```python
from build123d import *

# Parameters (mm, degrees)
F1_DEPTH = 3
F2_D     = 4


with BuildPart() as f1:
    # F0 (on Top) → F1 (new body)
    with BuildSketch(Plane.XY):
        Polygon((-13.5, -20), (13.5, -20), (13.5, 20), (-13.5, 20), (-13.5, 0), (-55, 0), (-55, -4.7585600987), (-55, -20), align=None)
    extrude(amount=F1_DEPTH)

    # F2 (through all)
    with Locations(Plane(origin=(0, 0, 0), x_dir=(1, 0, 0), z_dir=(0, 0, -1))):
        with Locations((-51, 10), (-26, 10), (-10, 10), (10, -10), (10, 10), (-10, -10)):
            Hole(F2_D / 2)


solid = f1.part
```
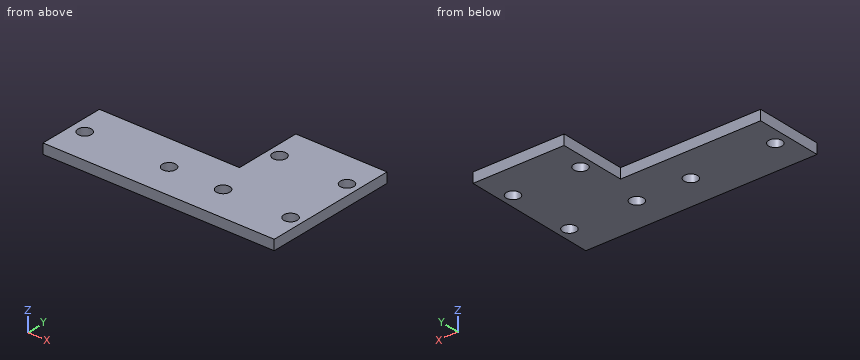
Work out the finished part from the listing and answer in its coordinate system (mm). Give positions to 0.01 mm unless a question says otherwise; leave off trailing zeros. Loops run counter-clockwise (first coordinate to the right, second up) from the corner with the lowest first, then second, coordinate; pieces in that order, holes last. Notation, with made-up numbers: M 2,-7 L 48,-7 A14 cw 48,-2 Z; hole C -12,-19.75 d4. An arc over 180 degrees is marked long. One line per item, written item: value. Start each with the question number.
1. Find section B-B (y = -10). Give the vertices of the cut face in (x, z).
2. Find section C-C (x = -51). Give the vertices of the cut face in (y, z), and give its area (3 significant figures).
3. Find the intervals of material crossed by probe 1 along X at (y, z) = (-10, 1); probe 2 along Y at (x, z) = (-10, 1.05); probe 3 along X at (y, z) = (10, 1.7), in increasing order.
4. Find section D-D (z = 1.7). Give the vertices of the cut face in (x, y), and give its area (3 significant figures).
5. Each of these flat-tipped pins is pushed along its axis until it touches: P1, Ø1.5, axis at y = 11.5, z = 1, coming from the -X side; P2, Ø0.9, axis at x = -38.5, z = 2, coming from the +Y side. Where does it stop, or does it pass through?
6. Find section A-A (x = -10). Give the vertices of the cut face in (y, z), and give its area (3 significant figures).
Reported:
1. outline: M -55,0 L -53,0 L -53,3 L -55,3 Z; M -49,0 L -28,0 L -28,3 L -49,3 Z; M -24,0 L -12,0 L -12,3 L -24,3 Z; M -8,0 L 8,0 L 8,3 L -8,3 Z; M 12,0 L 13.5,0 L 13.5,3 L 12,3 Z
2. outline: M -20,0 L -12,0 L -12,3 L -20,3 Z; M -8,0 L 0,0 L 0,3 L -8,3 Z
2. area: 48.0 mm²
3. probe 1: x = -55 to -53, -49 to -28, -24 to -12, -8 to 8, 12 to 13.5
3. probe 2: y = -20 to -12, -8 to 8, 12 to 20
3. probe 3: x = -13.5 to -12, -8 to 8, 12 to 13.5
4. outline: M -55,-20 L 13.5,-20 L 13.5,20 L -13.5,20 L -13.5,0 L -55,0 Z; hole C -51,-10 d4; hole C -26,-10 d4; hole C -10,-10 d4; hole C -10,10 d4; hole C 10,-10 d4; hole C 10,10 d4
4. area: 1,830 mm²
5. P1: stops at x = -13.5
5. P2: stops at y = 0
6. outline: M -20,0 L -12,0 L -12,3 L -20,3 Z; M -8,0 L 8,0 L 8,3 L -8,3 Z; M 12,0 L 20,0 L 20,3 L 12,3 Z
6. area: 96.0 mm²
